Geometry: final body of the model. Coordinates: model frame, mm. Give positions to 0.01 mm unless a question says otherwise; leave off trailing zeros. Loops run counter-clockwise (first coordinate to the right, second up) from the corner with the lowest first, then second, coordinate; pieces in that order, holes last. Notation, with made-up numbers: (-11, -13.5) - (-3, -13.5) arc R14 cw to (-3, 6.5) - close; hole circle Ø1 at (-16, -8). An arc over 180 degrees is marked (long way). Answer in a Markdown table with one row per item.
from build123d import *

# Parameters (mm, degrees)
F1_DEPTH = 1240
F3_D     = 5


with BuildPart() as f1:
    # F0 (on Top) → F1 (new body)
    with BuildSketch(Plane.XY):
        with BuildLine():
            Line((0, 19.5), (0, 0))
            Line((0, 0), (20, 0))
            Line((20, 0), (20, 20))
            Line((20, 20), (0.5, 20))
            ThreePointArc((0.5, 20), (0.146447, 19.853553), (0, 19.5))
        make_face()
        with BuildLine():
            ThreePointArc((1.5, 18), (1.646447, 18.353553), (2, 18.5))
            Line((2, 18.5), (18, 18.5))
            ThreePointArc((18, 18.5), (18.353553, 18.353553), (18.5, 18))
            Line((18.5, 18), (18.5, 2))
            ThreePointArc((18.5, 2), (18.353553, 1.646447), (18, 1.5))
            Line((18, 1.5), (2, 1.5))
            ThreePointArc((2, 1.5), (1.646447, 1.646447), (1.5, 2))
            Line((1.5, 2), (1.5, 18))
        make_face(mode=Mode.SUBTRACT)
    extrude(amount=F1_DEPTH)

    # F3 (through all)
    with Locations(Plane.XZ):
        with Locations((5, 1000), (15, 995), (5, 760), (15, 755), (5, 520), (15, 515), (5, 280), (15, 275)):
            Hole(F3_D / 2)


solid = f1.part
Q1. Material intervals for line 1 along Z through (x, y) = (15, 18.8); line 2 along Y through (x, z) = (4.25, 375.5), sorted ascending.
Check values:
| item | result |
|---|---|
| line 1 | 0 to 272.5, 277.5 to 512.5, 517.5 to 752.5, 757.5 to 992.5, 997.5 to 1240 |
| line 2 | 0 to 1.5, 18.5 to 20 |
Q2. Cut plane B-B (z = 979). Output: boundary loops of the cut face in (x, y).
Check values:
| item | result |
|---|---|
| outline | (0, 0) - (20, 0) - (20, 20) - (0.5, 20) arc R0.5 ccw to (0, 19.5) - close; hole (1.5, 2) arc R0.5 ccw to (2, 1.5) - (18, 1.5) arc R0.5 ccw to (18.5, 2) - (18.5, 18) arc R0.5 ccw to (18, 18.5) - (2, 18.5) arc R0.5 ccw to (1.5, 18) - close |
Q3. Cut plane A-A (y = 5.75). Output: boundary loops of the cut face in (x, z), and give its area (3 significant figures).
Check values:
| item | result |
|---|---|
| outline | (0, 0) - (1.5, 0) - (1.5, 1240) - (0, 1240) - close; (18.5, 0) - (20, 0) - (20, 1240) - (18.5, 1240) - close |
| area | 3,720 mm² |
